The model under review builds one solid part; all positions refer to its coordinate system, in mm. A direction names the side the tool comes from. Coordinates: 2 decimals unless noted, no trailing zeros. Order: outer loops, then holes, each group sorted by start corner. A loop starts at its lowest first (then second) coordinate and runs counter-clockwise, first axis right, second up. Notation, with made-up numbers: M -15.5,-15 L 38.5,-15 A22 cw 38.5,10 Z; hole C -3.5,30 d8. An arc over 180 degrees is marked long. Answer as CSV lines item,"result". Start each with the question number.
Q1. Machinability: for faces 1 (the face through (-32.5, 3, 60)), 2 (the face through (1, 6, -46)), which of the approach directions +Z, -Z, +X, -X, +Y, -Y give a long, thin tool a straight path to every point of the face, cutting with its end or side? Answer none if there is none.
Q2. For P1, Ø3.5, axis at x = 44, z = 0, coming from the +Y side; P2, Ø3, axis at y = 4, z = 65, coming from the -X side; P3, Ø3, axis at x = 15.5, y = 4.5, coming from the -Z side; P4, Ø1.8, axis at y = 2.5, z = -71, coming from the -X side, all flat-tipped, find the tip position at first contact; note any pin that passes through.
Q3. Consider section D-D on x = -35. Write out the cut boundary in (y, z), and give its area (3 significant figures).
Q4. Consider section C-C on z = -30. Write out the cut boundary in (x, y).
Q5. The part is to be moulded in two halves that separate along X. For faces 3 (the face through (61.198, 3.042, 44.282)), 4 (the face through (30.04, 2.96, 95.38)), 5 (the face through (1, 0, -46)), say which applies: +X half, -X half, draft (parallel to the pull), parting line (faces both ways), or undercut.
Q6. Wall thickness on L1, parallel to X at y = 4.75, z = 0; L2, parallel to Z at x = -14.5, y = 1.2; L3, parallel to X at y = 3.5, z = -67: over which ranges is each line inside the solid? List them lowest first. Write a range as [from, to].
Q7. Consider section B-B on y = 4.4. State how many separate pieces and enclosed holes the cut face has, and give its area (3 significant figures).
Q8. Consider section A-A on x = 0. Write out the cut boundary in (y, z), and give its area (3 significant figures).
from build123d import *

# Parameters (mm, degrees)
SKETCH2_R           = 100
BOSS_EXTRUDE1_DEPTH = 6
SKETCH3_W           = 0.5
SKETCH3_H           = 20
CUT_EXTRUDE1_DEPTH  = 142.548578234
SKETCH4_R           = 38.5
CUT_EXTRUDE2_DEPTH  = 142.548578234
SKETCH5_R           = 1.6
CUT_EXTRUDE3_DEPTH  = 142.548578234
SKETCH6_W           = 65
SKETCH6_H           = 30
CUT_EXTRUDE4_DEPTH  = 142.548578234


with BuildPart() as part:
    # Sketch2 → Boss-Extrude1 (new body)
    with BuildSketch(Plane(origin=(0, 0, 0), x_dir=(1, 0, 0), z_dir=(0, 1, 0))):
        with Locations(Location((0, 0, 0), (0, 0, 270))):
            Circle(SKETCH2_R)
    extrude(amount=BOSS_EXTRUDE1_DEPTH)

    # Sketch3 → Cut-Extrude1 (cut, through all)
    with BuildSketch(Plane(origin=(0, 6, 0), x_dir=(1, 0, 0), z_dir=(0, 1, 0))):
        with Locations((-7.5, 75)):
            Rectangle(SKETCH3_W, SKETCH3_H)
        with Locations((7.5, 75)):
            Rectangle(SKETCH3_W, SKETCH3_H)
        Polygon((60.166651246, -25.788303121), (77.487159322, -35.788303121), (77.237159322, -36.221315823), (59.916651246, -26.221315823), align=None)
        Polygon((52.666651246, -38.778684177), (69.987159322, -48.778684177), (69.737159322, -49.211696879), (52.416651246, -39.211696879), align=None)
        Polygon((-52.416651246, -39.211696879), (-69.737159322, -49.211696879), (-69.987159322, -48.778684177), (-52.666651246, -38.778684177), align=None)
        Polygon((-59.916651246, -26.221315823), (-77.237159322, -36.221315823), (-77.487159322, -35.788303121), (-60.166651246, -25.788303121), align=None)
    extrude(amount=-CUT_EXTRUDE1_DEPTH, mode=Mode.SUBTRACT)

    # Sketch4 → Cut-Extrude2 (cut, through all)
    with BuildSketch(Plane(origin=(0, 6, 0), x_dir=(1, 0, 0), z_dir=(0, 1, 0))):
        with Locations(Location((0, 0, 0), (0, 0, 270))):
            Circle(SKETCH4_R)
    extrude(amount=-CUT_EXTRUDE2_DEPTH, mode=Mode.SUBTRACT)

    # Sketch5 → Cut-Extrude3 (cut, through all)
    with BuildSketch(Plane(origin=(0, 6, 0), x_dir=(1, 0, 0), z_dir=(0, 1, 0))):
        with Locations(Location((-44, 0, 0), (0, 0, 270))):
            Circle(SKETCH5_R)
        with Locations(Location((44, 0, 0), (0, 0, 270))):
            Circle(SKETCH5_R)
    extrude(amount=-CUT_EXTRUDE3_DEPTH, mode=Mode.SUBTRACT)

    # Sketch6 → Cut-Extrude4 (cut, through all)
    with BuildSketch(Plane(origin=(0, 6, 0), x_dir=(1, 0, 0), z_dir=(0, 1, 0))):
        with Locations((0, -60)):
            Rectangle(SKETCH6_W, SKETCH6_H)
    extrude(amount=-CUT_EXTRUDE4_DEPTH, mode=Mode.SUBTRACT)


solid = part.part
Evaluation:
1,face 1,"+Y, -Y"
1,face 2,"+Z, -Z, +X, -X, +Y"
2,P1,"stops at y = 6"
2,P2,"stops at x = -77.25"
2,P3,"stops at z = -99.02"
2,P4,"stops at x = -71.32"
3,outline,"M 0,-93.67 L 6,-93.67 L 6,-16.04 L 0,-16.04 Z; M 0,16.04 L 6,16.04 L 6,93.67 L 0,93.67 Z"
3,area,"932 mm²"
4,outline,"M -95.39,0 L -24.13,0 L -24.13,6 L -95.39,6 Z; M 24.13,0 L 95.39,0 L 95.39,6 L 24.13,6 Z"
5,face 3,"undercut"
5,face 4,"parting line"
5,face 5,"draft"
6,L1,"x = [-100, -45.6], [-42.4, -38.5], [38.5, 42.4], [45.6, 100]"
6,L2,"z = [-98.94, -35.67], [35.67, 45], [75, 98.94]"
6,L3,"x = [-74.24, -7.75], [-7.25, 7.25], [7.75, 74.24]"
7,separate pieces,"1"
7,enclosed holes,"10"
7,area,"24,700 mm²"
8,outline,"M 0,-100 L 6,-100 L 6,-38.5 L 0,-38.5 Z; M 0,38.5 L 6,38.5 L 6,45 L 0,45 Z; M 0,75 L 6,75 L 6,100 L 0,100 Z"
8,area,"558 mm²"
